Can you work these out from the model? Positions are in its coordinate system, mm. Round coordinates to 2 decimals unless told otherwise and drop trailing zeros. Write each loop counter-clockwise with the first axis right and the second up, starting at its lowest first coordinate (ties: lowest second). Pieces come first, ordered by that corner, then holes.
Q1. Please list where these lines run through material, in increasing order: line 1 along Z through (x, y) = (19.5, 4.2); line 2 along Z through (x, y) = (-25, 2.75); line 3 along X through (y, z) = (6, -18).
Q2. If we section it at C-C (y = 3): Give the number of separate pieces and of enclosed holes in the cut face, plus the area to 3 significant figures.
Q3. If we section it at A-A (x = 0): Please give me the cut outline in (y, z).
Q4. I'm going to push flat-ended pins straight in: pin 1 Ø6 at (x, z) = (-19.5, 27) entering from -Y; pin 2 Ø2 at (x, z) = (19.5, 27) entering from +Y; pin 3 Ø10 at (x, z) = (11.5, 22.5) entering from -Y. Where does each tip first touch, or does it pass through?
Q5. If we section it at B-B (z = -10): Please give me the cut outline in (x, y), plus the area to 3 significant figures.
Q6. If we section it at D-D (x = 24): Please give me the cut outline in (y, z).
Solid Edge part; units mm, degrees
sketch "Sketch1" plane through (0, 0, 0) normal (0, -1, 0) x (1, 0, 0)
  circle A0 centre (0, 0) radius 29
  line L0 (31, 31) -> (-31, 31)
  line L1 (-31, 31) -> (-31, -31)
  line L2 (-31, -31) -> (31, -31)
  line L3 (31, 31) -> (31, -31)
  dimension "D1" = 31
  dimension "D2" = 31
extrude "Protrusion1" add sketch "Sketch1" against normal blind 7
hole "Bohrung_17" at (-25, 0, 25) direction (0, 1, 0) diameter 4 end up to next
hole "Hole1" at (25, 0, 25) direction (0, 1, 0) diameter 4 end up to next
hole "Hole2" at (25, 0, -25) direction (0, 1, 0) diameter 4 end up to next
hole "Hole3" at (-25, 0, -25) direction (0, 1, 0) diameter 4 end up to next
hole "Bohrung_21" at (-19.5, 0, 27) direction (0, 1, 0) diameter 3.6 end up to next countersink diameter 6.5 countersink angle 90
hole "Hole4" at (19.5, 0, 27) direction (0, 1, 0) diameter 3.6 end up to next countersink diameter 6.5 countersink angle 90
hole "Hole5" at (19.5, 0, -27) direction (0, 1, 0) diameter 3.6 end up to next countersink diameter 6.5 countersink angle 90
hole "Hole6" at (-19.5, 0, -27) direction (0, 1, 0) diameter 3.6 end up to next countersink diameter 6.5 countersink angle 90
fillet "Verrundung_1" radius 5 4 edges at (31, 3.5, -31) (-31, 3.5, -31) (-31, 3.5, 31) (31, 3.5, 31)
properties part number "42" material "Polyacticacid"
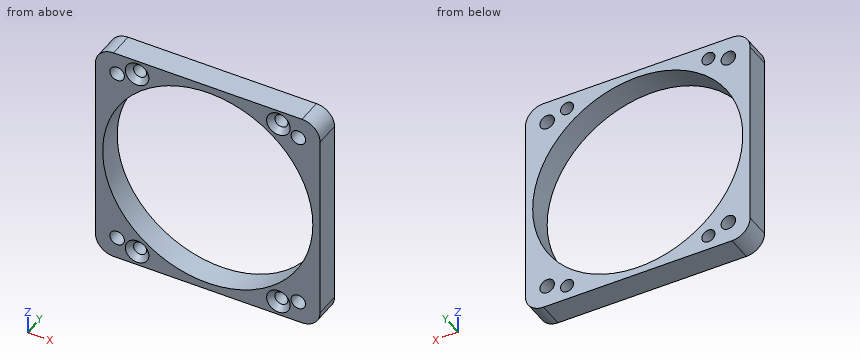
A:
1. line 1: z = -31 to -28.8, -25.2 to -21.47, 21.47 to 25.2, 28.8 to 31
1. line 2: z = -31 to -27, -23 to -14.7, 14.7 to 23, 27 to 31
1. line 3: x = -31 to -22.74, 22.74 to 31
2. separate pieces: 1
2. enclosed holes: 9
2. area: 1,090 mm2
3. outline: (0, -31) - (7, -31) - (7, -29) - (0, -29) - close; (0, 29) - (7, 29) - (7, 31) - (0, 31) - close
4. pin 1: stops at y = 0.25
4. pin 2: passes through
4. pin 3: stops at y = 0
5. outline: (-31, 0) - (-27.22, 0) - (-27.22, 7) - (-31, 7) - close; (27.22, 0) - (31, 0) - (31, 7) - (27.22, 7) - close
5. area: 52.9 mm2
6. outline: (0, -31) - (7, -31) - (7, -26.73) - (0, -26.73) - close; (0, -23.27) - (7, -23.27) - (7, -16.28) - (0, -16.28) - close; (0, 16.28) - (7, 16.28) - (7, 23.27) - (0, 23.27) - close; (0, 26.73) - (7, 26.73) - (7, 31) - (0, 31) - close
